```python
from build123d import *

# Parameters (mm, degrees)
CROQUIS1_R              = 23.5
SALIENTE_EXTRUIR1_DEPTH = 0.5
CROQUIS2_R              = 21.5
SALIENTE_EXTRUIR2_DEPTH = 13
CROQUIS3_R              = 4.05
CORTAR_EXTRUIR1_DEPTH   = 40


with BuildPart() as part:
    # Croquis1 → Saliente-Extruir1 (new, symmetric)
    with BuildSketch(Plane.XY):
        Circle(CROQUIS1_R)
    extrude(amount=SALIENTE_EXTRUIR1_DEPTH, both=True)

    # Croquis2 → Saliente-Extruir2 (add)
    with BuildSketch(Plane.XY.offset(0.5)):
        with Locations(Location((0, 0, 0), (0, 0, 180))):
            Circle(CROQUIS2_R)
    extrude(amount=SALIENTE_EXTRUIR2_DEPTH)

    # Croquis3 → Cortar-Extruir1 (cut)
    with BuildSketch(Plane.XY.offset(13.5)):
        Circle(CROQUIS3_R)
    extrude(amount=-CORTAR_EXTRUIR1_DEPTH, mode=Mode.SUBTRACT)


solid = part.part
```
Input: part model. Units: mm. Frame: model coordinates. A direction names the side the tool comes from. Coordinates: 2 decimals unless noted, no trailing zeros. Write each loop counter-clockwise with the first axis right and the second up, starting at its lowest first coordinate (ties: lowest second). Pieces come first, ordered by that corner, then holes. Notation, with made-up numbers: (36, 45) -> (63, 45) arc R33 cw to (63, 81) -> close; hole circle Ø3 at (71, 80.5). An arc over 180 degrees is marked (long way). Answer as a JSON object with one key per item and string values.
1. Access query for faces 4 (the face through (0, -5, -0.5)), 5 (the face through (10.33, -19.04, 0.5)). Directions: +Z, -Z, +X, -X, +Y, -Y. A direction counts if a zero-diameter tool reaches every point of the face in a straight line with its end or side. Return the directions, or none.
Result set:
{"face 4": "-Z, +X, -X, +Y, -Y", "face 5": "+Z"}
2. Section D-D on z = 4.25. Return the cut outline in (x, y).
Result set:
{"outline": "circle Ø43 at (0, 0); hole circle Ø8.1 at (0, 0)"}
3. Section C-C on y = -10. Return the cut outline in (x, z), then the cut area to 3 significant figures.
Result set:
{"outline": "(-21.27, -0.5) -> (21.27, -0.5) -> (21.27, 0.5) -> (19.03, 0.5) -> (19.03, 13.5) -> (-19.03, 13.5) -> (-19.03, 0.5) -> (-21.27, 0.5) -> close", "area": "537 mm2"}
4. Mould query, pull axis X, two halves, no side actions, for faces 1 (the face through (2.799, -21.317, 6.909)), 2 (the face through (-0.878, -3.954, 6.598)), 3 (the face through (-4.5, -0.3, 13.5)). Classes: released by +X, released by -X, zero draft, split by the parting line, or undercut.
Result set:
{"face 1": "split by the parting line", "face 2": "undercut", "face 3": "zero draft"}
5. Section A-A on x = 0. Return the cut outline in (y, z), then the cut area to 3 significant figures.
Result set:
{"outline": "(-23.5, -0.5) -> (-4.05, -0.5) -> (-4.05, 13.5) -> (-21.5, 13.5) -> (-21.5, 0.5) -> (-23.5, 0.5) -> close; (4.05, -0.5) -> (23.5, -0.5) -> (23.5, 0.5) -> (21.5, 0.5) -> (21.5, 13.5) -> (4.05, 13.5) -> close", "area": "493 mm2"}
6. First-contact query: P1, Ø1.5, axis at x = 4, z = 6, coming from the +Y side; P2, Ø5, axis at y = -5, z = 7.5, coming from the +X side; P3, Ø2, axis at x = 2.5, z = 1, coming from the -Y side; P4, Ø13, axis at x = 0, y = 0, coming from the -Z side. Flat tips, straight axial feed; report the tip coordinate or a pass-through.
Result set:
{"P1": "stops at y = 21.25", "P2": "stops at x = 21.35", "P3": "stops at y = -23.44", "P4": "stops at z = -0.5"}
7. Material intervals for line 1 (Y direction, x = 0, z = 10); line 2 (Z direction, x = -13.5, y = -18); line 3 (X direction, y = 2.5, z = 9.75), sorted ascending. Write a range as from..to.
Result set:
{"line 1": "y = -21.5..-4.05, 4.05..21.5", "line 2": "z = -0.5..0.5", "line 3": "x = -21.35..-3.19, 3.19..21.35"}
